The figure shows three views and two pictorial views of one solid part (mm, origin at its lowest corner). Answer the questions. A direction names the side the tool comes from. Give positions to 0.01 mm unless a question says otherwise; leave off trailing zeros. Order: outer loops, then holes, each group sorted by start corner. A loop starts at its lowest first (then second) coordinate and runs counter-clockwise, first axis right, second up. Notation, with made-up numbers: M 72.5,34.25 L 128.5,34.25 A8 cw 128.5,49.25 Z; hole C -33.75,28 d1. An arc over 180 degrees is marked long. One line per item, written item: value. Start each with the question number.
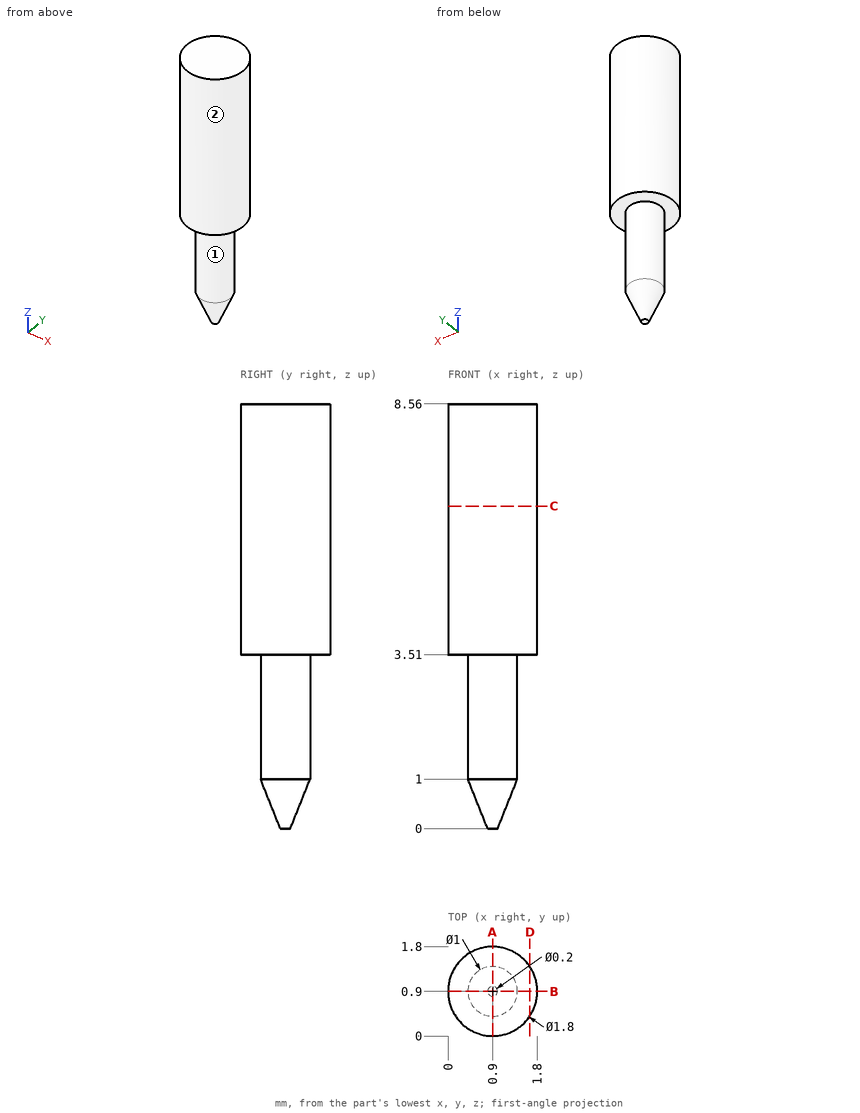
Q1. This flat-tipped pin is pushed along its axis until it touches: pin 1 (1 mm diameter, centred on y = 1.5, z = 2, fed in from -X). Where does it stop, or does it pass through?
Q2. Find section A-A, the plane x = 0.9. Give the vertices of the cut face in (y, z), then the cut area to 3 significant figures.
Q3. Consider probe 1 along Y at (x, z) = (0.85, 2); probe 2 along Z at (x, y) = (1.55, 1.35); probe 3 along Y at (x, z) = (0.6, 7.25). Determine where each line is inside the solid, lowest interval first.
Q4. A tool of negligible diameter and unlimited length cuts with its end or side. For the marked faces 1 and 2, from which of +Z, -Z, +X, -X, +Y, -Y can it reach the whole face along a straight path? Write none if from no direction.
Q5. Find section C-C, the plane z = 6.5. Give the vertices of the cut face in (x, y), then the cut area to 3 significant figures.
Q6. Find section D-D, the plane x = 1.65. Give the vertices of the cut face in (y, z).
Evaluation:
1. pin 1: x = 0.41
2. outline: M 0,3.51 L 0.4,3.51 L 0.4,1 L 0.8,0 L 1,0 L 1.4,1 L 1.4,3.51 L 1.8,3.51 L 1.8,8.56 L 0,8.56 Z
2. area: 12.2 mm2
3. probe 1: 0.4 to 1.4
3. probe 2: 3.51 to 8.56
3. probe 3: 0.05 to 1.75
4. face 1: -Z
4. face 2: +Z, -Z
5. outline: C 0.9,0.9 d1.8
5. area: 2.54 mm2
6. outline: M 0.4,3.51 L 1.4,3.51 L 1.4,8.56 L 0.4,8.56 Z
